Geometry check sheet. Reference: the model listing, model coordinates, mm. A direction names the side the tool comes from. Coordinates: 2 decimals unless noted, no trailing zeros. Loops run counter-clockwise (first coordinate to the right, second up) from the corner with the lowest first, then second, coordinate; pieces in that order, holes last. Notation, with made-up numbers: (37.5, 19.25) - (45.5, 19.25) arc R32 cw to (45.5, 45.25) - close; hole circle Ø6 at (21, 32.5). An arc over 180 degrees is marked (long way). One line per item, written item: value.
from build123d import *

# Parameters (mm, degrees)
F2_DEPTH = 150


with BuildPart() as f2:
    # F1 (on Right) → F2 (new body, through all)
    with BuildSketch(Plane.YZ):
        Polygon((-234.807621, 0), (-259.807621, 0), (-259.807621, -2), (-236.807621, -2), (-236.807621, -25), (-234.807621, -25), align=None)
    extrude(amount=F2_DEPTH)

    # F3: F2 across plane


with BuildPart() as f2_1:
    add(f2.part)
    add(f2.part.mirror(Plane.YZ))


solid = f2_1.part
(1) Access from +Z, -Z, +X, -X, +Y, -Y to the whole of each face (thin tool, end or side, straight path). Record for faces 1 (the face through (2, -236.808, -13)), 2 (the face through (-150, -242, -1)).
Reply:
face 1: -Z, +X, -X, -Y
face 2: +Z, -Z, -X, +Y, -Y
(2) Cross-section at A-A on x = -34. Record the cut outline in (y, z).
Reply:
outline: (-259.81, -2) - (-236.81, -2) - (-236.81, -25) - (-234.81, -25) - (-234.81, 0) - (-259.81, 0) - close
(3) Material ranges on probe 1 along Z at (x, y) = (-107, -251.5); probe 2 along Y at (x, z) = (22.5, -3.25), recorded low to high. Write a range as from..to.
Reply:
probe 1: -2..0
probe 2: -236.81..-234.81
(4) Go/stop test with flat-tipped pins: pin 1 Ø5 at (x, z) = (-92.5, -5) entering from -Y; pin 2 Ø7 at (x, y) = (-13.5, -246.5) entering from -Z. Record where each tip stops, or that it passes through.
Reply:
pin 1: y = -236.81
pin 2: z = -2
(5) Cross-section at C-C on y = -248. Record the cut outline in (x, z).
Reply:
outline: (-150, -2) - (150, -2) - (150, 0) - (-150, 0) - close
(6) Cross-section at B-B on z = -17.25. Record the cut outline in (x, y).
Reply:
outline: (-150, -236.81) - (150, -236.81) - (150, -234.81) - (-150, -234.81) - close
